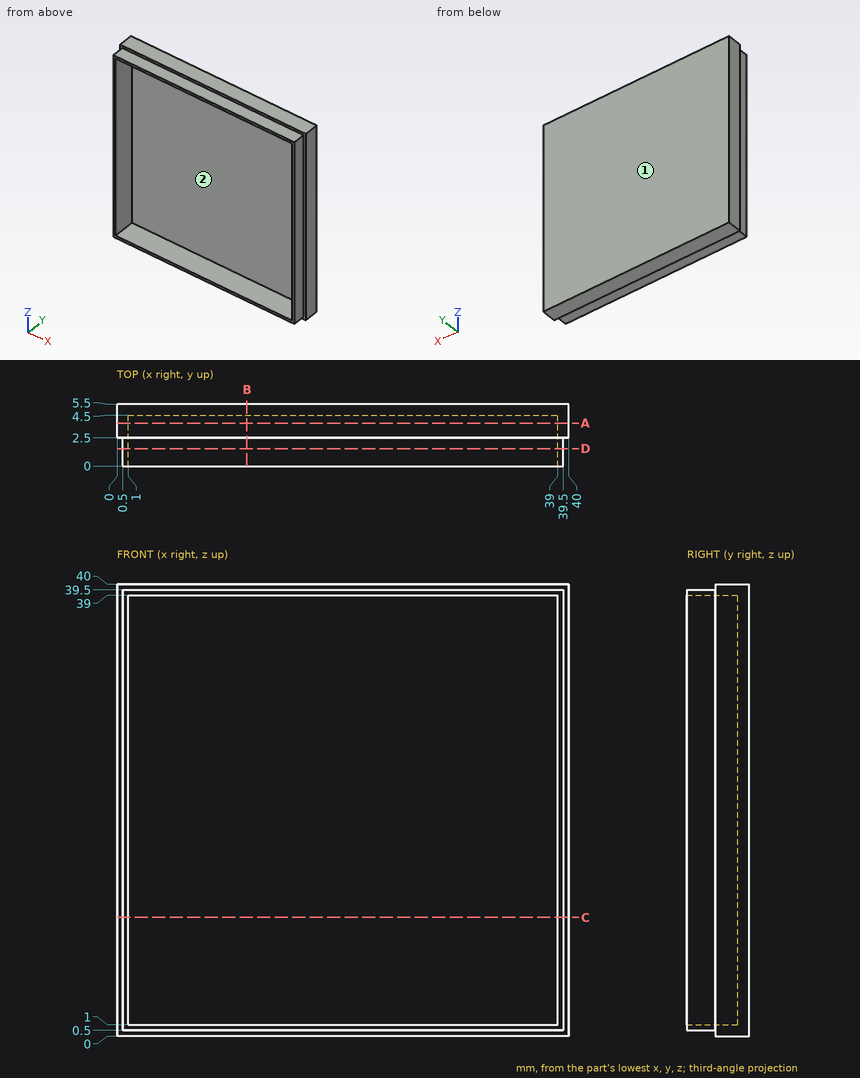
Here's the drawing with two shaded views (mm, measured from the low corner). I have some questions. Give positions to 0.01 mm unless a question says otherwise; leave off trailing zeros. Order: outer loops, then holes, each group sorted by start corner. A loop starts at its lowest first (then second) coordinate and runs counter-clockwise, first axis right, second up. Notation, with made-up numbers: (53.25, 85) -> (95.25, 85) arc R24 ccw to (95.25, 118) -> close; hole circle Ø8 at (36.5, -10.5). An arc over 180 degrees is marked (long way). One line per item, written item: value. Start each with the question number.
1. Imagine slicing it at A-A, the plane y = 3.8. List the corners of the cut face in (x, z) for me.
2. Imagine slicing it at D-D, the plane y = 1.55. List the corners of the cut face in (x, z) for me, plus the area to 3 significant figures.
3. Imagine slicing it at C-C, the plane z = 10.5. List the corners of the cut face in (x, y) for me.
4. Imagine slicing it at B-B, the plane x = 11.5. List the corners of the cut face in (y, z) for me.
5. I need wall thicknesses on probe 1 along Z at (x, y) = (31, 2); probe 2 along Z at (x, y) = (9, 3.7). Which ranges of each line are inside material? Lowest first, please. Write a range as from..to.
6. We'd pull the mould along X, two halves only. Please class the marked faces 1 and 2: released by +X, released by -X, zero draft, split by the parting line, or undercut.
7. Will these pins go through, and if not, where does the flat tip stop? pin 1 Ø1.2 at (x, y) = (20, 1.5) entering from -Z; pin 2 Ø1.2 at (y, z) = (1, 18) entering from -X; pin 3 Ø0.8 at (x, y) = (12.5, 1) entering from +Z.
Values follow:
1. outline: (0, 0) -> (40, 0) -> (40, 40) -> (0, 40) -> close; hole (1, 1) -> (39, 1) -> (39, 39) -> (1, 39) -> close
2. outline: (0.5, 0.5) -> (39.5, 0.5) -> (39.5, 39.5) -> (0.5, 39.5) -> close; hole (1, 1) -> (39, 1) -> (39, 39) -> (1, 39) -> close
2. area: 77.0 mm2
3. outline: (0, 2.5) -> (0.5, 2.5) -> (0.5, 0) -> (1, 0) -> (1, 4.5) -> (39, 4.5) -> (39, 0) -> (39.5, 0) -> (39.5, 2.5) -> (40, 2.5) -> (40, 5.5) -> (0, 5.5) -> close
4. outline: (0, 0.5) -> (2.5, 0.5) -> (2.5, 0) -> (5.5, 0) -> (5.5, 40) -> (2.5, 40) -> (2.5, 39.5) -> (0, 39.5) -> (0, 39) -> (4.5, 39) -> (4.5, 1) -> (0, 1) -> close
5. probe 1: z = 0.5..1, 39..39.5
5. probe 2: z = 0..1, 39..40
6. face 1: zero draft
6. face 2: undercut
7. pin 1: stops at z = 0.5
7. pin 2: stops at x = 0.5
7. pin 3: stops at z = 39.5
